Build history of the part. All positions in model axes, mm. Face numbers are marked on the shaded views. A direction names the side the tool comes from. Give positions to 0.01 mm unless a question says otherwise; leave off trailing zeros. Loops run counter-clockwise (first coordinate to the right, second up) from the corner with the lowest first, then second, coordinate; pieces in that order, holes last. Notation, with made-up numbers: M -37,56 L 4,56 A18 ccw 4,91 Z; hole C 36.5,-4.5 d9. An arc over 180 degrees is marked long. Answer as a JSON object with one key per item and string values. Group by question number.
1. Slice it at C-C (z = 5). List the corners of the cut face in (x, y).
2. Mould opens along Z. For the marked faces 1, 2 and 3 say: released by +Z, released by -Z, zero draft, split by the parting line, or undercut.
3. Slice it at B-B (x = -28). List the corners of the cut face in (y, z), then the cut area to 3 significant figures.
4. Drop flat-ended pins along their axis: pin 1 Ø15 at (x, y) = (0, 45) entering from +Z; pin 2 Ø8 at (x, y) = (-28, 78) entering from +Z; pin 3 Ø3.5 at (x, z) = (-6.5, 4.5) entering from +Y. Give the stop position or say it passes through.
5. 3-axis set-ups, long thin cutter, end or side, ignore diameter. For the marked faces 4, 5 and 6: which of +Z, -Z, +X, -X, +Y, -Y reach the whole face in a straight line?
6. Drill centre lines: line 1 along Y through (x, z) = (28, 3); line 2 along X through (y, z) = (80, 11.25); line 3 along X through (y, z) = (45.5, 8.25). Where is each one in solid material? Low to high. Write a range as [from, to].
7. Slice it at D-D (y = 13). List the corners of the cut face in (x, z), then the cut area to 3 significant figures.
8. Slice it at A-A (x = 0). List the corners of the cut face in (y, z), then the cut area to 3 significant figures.
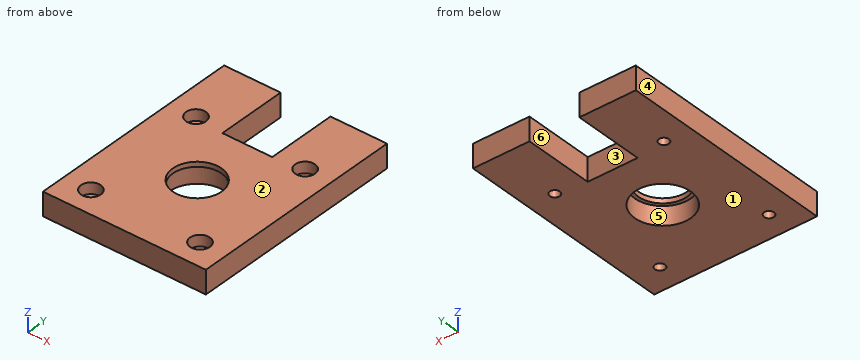
from build123d import *

# Parameters (mm, degrees)
SKETCH_R        = 2.54
PAD_DEPTH       = 12
SKETCH001_R     = 14.35
POCKET_DEPTH    = 9.53
SKETCH002_R     = 12.5
POCKET001_DEPTH = 12.001
SKETCH003_R     = 5.08
POCKET002_DEPTH = 5.65


with BuildPart() as part:
    # Sketch → Pad (new body)
    with BuildSketch(Plane.XY):
        Polygon((0, 0), (-41.8, 0), (-41.8, 112), (-12.8, 112), (-12.8, 76), (0, 76), align=None)
        with Locations((-28, 13)):
            Circle(SKETCH_R, mode=Mode.SUBTRACT)
        with Locations((-28, 78)):
            Circle(SKETCH_R, mode=Mode.SUBTRACT)
    pad = extrude(amount=PAD_DEPTH)

    # Mirrored: Pad across Sketch V_Axis
    add(pad.mirror(Plane(origin=(0, 0, 0), x_dir=(0, 0, 1), z_dir=(1, 0, 0))))

    # Sketch001 → Pocket (cut)
    with BuildSketch(Plane.XY):
        with Locations((0, 45)):
            Circle(SKETCH001_R)
    extrude(amount=POCKET_DEPTH, mode=Mode.SUBTRACT)

    # Sketch002 → Pocket001 (cut, through all)
    with BuildSketch(Plane.XY):
        with Locations((0, 45)):
            Circle(SKETCH002_R)
    extrude(amount=POCKET001_DEPTH, mode=Mode.SUBTRACT)

    # Sketch003 (on Face5 of Pocket001) → Pocket002 (cut)
    with BuildSketch(Plane.XY.offset(12)):
        with Locations((-28, 13)):
            Circle(SKETCH003_R)
        with Locations((-28, 78)):
            Circle(SKETCH003_R)
        with Locations((28, 78)):
            Circle(SKETCH003_R)
        with Locations((28, 13)):
            Circle(SKETCH003_R)
    extrude(amount=-POCKET002_DEPTH, mode=Mode.SUBTRACT)


solid = part.part
Established:
{
 "1": {"outline": "M -41.8,0 L 41.8,0 L 41.8,112 L 12.8,112 L 12.8,76 L -12.8,76 L -12.8,112 L -41.8,112 Z; hole C -28,13 d5.08; hole C -28,78 d5.08; hole C 0,45 d28.7; hole C 28,13 d5.08; hole C 28,78 d5.08"},
 "2": {"face 1": "released by -Z", "face 2": "released by +Z", "face 3": "zero draft"},
 "3": {"outline": "M 0,0 L 10.46,0 L 10.46,6.35 L 7.92,6.35 L 7.92,12 L 0,12 Z; M 15.54,0 L 75.46,0 L 75.46,6.35 L 72.92,6.35 L 72.92,12 L 18.08,12 L 18.08,6.35 L 15.54,6.35 Z; M 80.54,0 L 112,0 L 112,12 L 83.08,12 L 83.08,6.35 L 80.54,6.35 Z", "area": "1,160 mm^2"},
 "4": {"pin 1": "passes through", "pin 2": "stops at z = 6.35", "pin 3": "stops at y = 76"},
 "5": {"face 4": "+Z, -Z, -X, +Y, -Y", "face 5": "-Z", "face 6": "+Z, -Z, +Y"},
 "6": {"line 1": "y = [0, 10.46], [15.54, 75.46], [80.54, 112]", "line 2": "x = [-41.8, -32.67], [-23.33, -12.8], [12.8, 23.33], [32.67, 41.8]", "line 3": "x = [-41.8, -14.34], [14.34, 41.8]"},
 "7": {"outline": "M -41.8,0 L -30.54,0 L -30.54,6.35 L -33.08,6.35 L -33.08,12 L -41.8,12 Z; M -25.46,0 L 25.46,0 L 25.46,6.35 L 22.92,6.35 L 22.92,12 L -22.92,12 L -22.92,6.35 L -25.46,6.35 Z; M 30.54,0 L 41.8,0 L 41.8,12 L 33.08,12 L 33.08,6.35 L 30.54,6.35 Z", "area": "824 mm^2"},
 "8": {"outline": "M 0,0 L 30.65,0 L 30.65,9.53 L 32.5,9.53 L 32.5,12 L 0,12 Z; M 57.5,9.53 L 59.35,9.53 L 59.35,0 L 76,0 L 76,12 L 57.5,12 Z", "area": "577 mm^2"}
}
